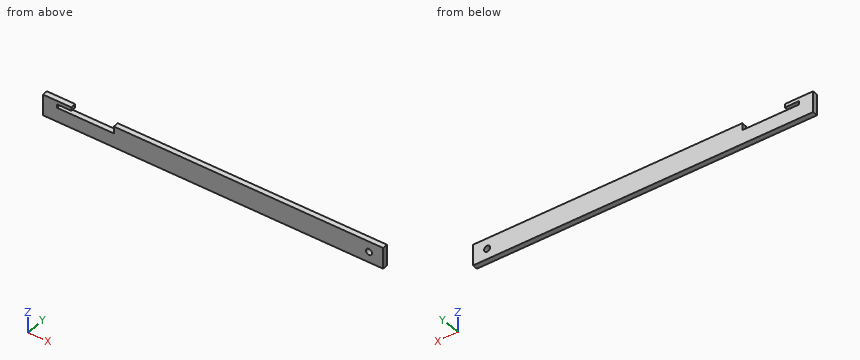
from build123d import *

# Parameters (mm, degrees)
F0_W     = 101.6
F0_H     = 44.45
F1_DEPTH = 6.35
F2_W     = 609.6
F2_H     = 38.1
F2_W_2   = 101.6
F2_H_2   = 6.35
F3_DEPTH = 9.525
F4_DEPTH = 9.525
F6_W     = 76.2
F6_H     = 25.4
F7_DEPTH = 25.4
F8_R     = 5.5
F9_DEPTH = 25.4


# Not quite as in the source:
# - ends of sketch curves that miss each other by under 0.0002 mm in the source are joined


with BuildPart() as f1:
    # F0 (on Top) → F1 (new body)
    with BuildSketch(Plane.XY):
        with Locations((-3.1162388623, -13.4853734154)):
            Rectangle(F0_W, F0_H)
    extrude(amount=F1_DEPTH)

    # F2 (on face) → F4 (cut)
    with BuildSketch(Plane.XZ.offset(35.7103734154)):
        with Locations((-3.1162388623, 3.175)):
            Rectangle(F2_W_2, F2_H_2)
    extrude(amount=-F4_DEPTH, mode=Mode.SUBTRACT)


with BuildPart() as f3:
    # F2 (on face) → F3 (new body)
    with BuildSketch(Plane.XZ.offset(35.7103734154)):
        with Locations((225.4837611377, -6.35)):
            Rectangle(F2_W, F2_H)
        with Locations((-3.1162388623, 3.175)):
            Rectangle(F2_W_2, F2_H_2, mode=Mode.SUBTRACT)
    extrude(amount=-F3_DEPTH)

    # F6 (on face) → F7 (cut)
    with BuildSketch(Plane.XZ.offset(35.7103734154)):
        with Locations((9.5837611377, 19.05)):
            Rectangle(F6_W, F6_H)
    extrude(amount=-F7_DEPTH, mode=Mode.SUBTRACT)

    # F8 (on face) → F9 (cut)
    with BuildSketch(Plane.XZ.offset(35.7103734154)):
        with Locations((504.8837611377, -6.35)):
            Circle(F8_R)
    extrude(amount=-F9_DEPTH, mode=Mode.SUBTRACT)


solid = f3.part
The model under review builds one solid part; all positions refer to its coordinate system, in mm. Round coordinates to 2 decimals unless told otherwise and drop trailing zeros. Loops run counter-clockwise (first coordinate to the right, second up) from the corner with the lowest first, then second, coordinate; pieces in that order, holes last. Notation, with made-up numbers: (89.25, 29) -> (114.25, 29) arc R23 ccw to (114.25, 51) -> close; hole circle Ø5 at (31, -14.5). An arc over 180 degrees is marked (long way). One line per question, with ' | ' between items. Start each with the question number.
Item 1: Add section B-B, the plane z = -6.35. Write out the cut boundary in (x, y).
Item 2: Add section A-A, the plane y = -32.25. Write out the cut boundary in (x, z).
Item 3: Wall thickness on line 1 along X through (y, z) = (-32.5, 1); line 2 along X through (y, z) = (-33.25, 7); line 3 along Z through (x, y) = (-52, -32.5): over which ranges is each line inside the solid? List them lowest first. Write a range as [from, to].
Item 4: For pin 1 (10 mm diameter, centred on x = 504.88, z = -6.35, fed in from -Y), flat-tipped, find the tip position at first contact; note if it passes through.
Return value:
1) outline: (-79.32, -35.71) -> (499.38, -35.71) -> (499.38, -26.19) -> (-79.32, -26.19) -> close; (510.38, -35.71) -> (530.28, -35.71) -> (530.28, -26.19) -> (510.38, -26.19) -> close
2) outline: (-79.32, -25.4) -> (530.28, -25.4) -> (530.28, 12.7) -> (47.68, 12.7) -> (47.68, 0) -> (-53.92, 0) -> (-53.92, 6.35) -> (-28.52, 6.35) -> (-28.52, 12.7) -> (-79.32, 12.7) -> close; hole circle Ø11 at (504.88, -6.35)
3) line 1: x = [-79.32, -53.92], [47.68, 530.28] | line 2: x = [-79.32, -28.52], [47.68, 530.28] | line 3: z = [-25.4, 0], [6.35, 12.7]
4) pin 1: passes through
